Could you check a few things on this model? Use its own coordinates, in mm. Coordinates: 2 decimals unless noted, no trailing zeros. Loops run counter-clockwise (first coordinate to the right, second up) from the corner with the lowest first, then second, coordinate; pieces in that order, holes last. Notation, with made-up numbers: (19, 9) - (23, 9) arc R22 ccw to (23, 39) - close; hole circle Ø4 at (21, 57). An arc over 180 degrees is marked (long way). One line per item, written item: value. Start each with the question number.
(1) If I drill on line 1 along X through (y, z) = (1.8, 0); line 2 along X through (y, z) = (0.4, 85); line 3 along Z through (x, y) = (176, 2.3), over which ranges is the centre line in solid material (lowest first)? Write a range as from..to.
(2) If we section it at B-B on z = -17: Write out the boundary of the cut face in (x, y).
(3) If we section it at A-A on y = 2.5: Write out the boundary of the cut face in (x, z).
(4) If we section it at C-C on z = 63: Write out the boundary of the cut face in (x, y).
(5) I'm going to push a flat-ended pin straight in: P1, Ø4, axis at x = 202, z = 0, coming from the -Y side. Where does the tip first touch, or does it pass through?
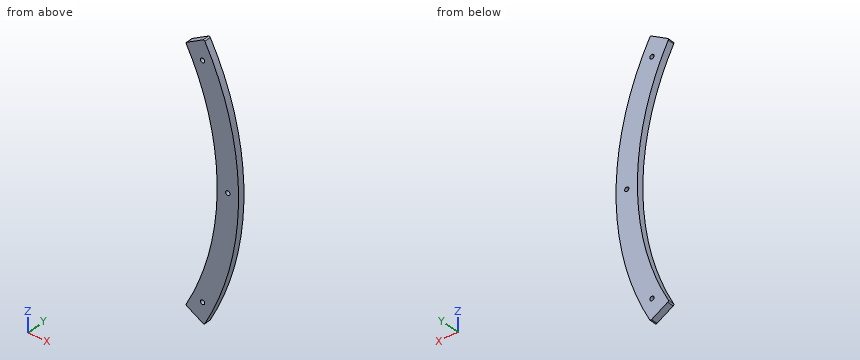
Autodesk Fusion 360 part; units mm, degrees
sketch "スケッチ1" plane through (0, 0, 0) normal (0, 1, 0) x (1, 0, 0)
  arc A0 (181.8653, -105) -> (181.8653, 105) centre (0, 0) ccw
  line L0 (181.8653, 105) -> (0, 0)
  line L1 (0, 0) -> (181.8653, -105)
  line L2 (0, 0) -> (210, 0)
  arc A1 (168.0089, -97) -> (168.0089, 97) centre (0, 0) ccw
  line L3 (10, 0) -> (184.3138, 100.6401)
  line L4 (10, 0) -> (184.3138, -100.6401)
  arc A2 (183.0742, -85.3689) -> (183.0742, 85.3689) centre (0, 0) ccw
  line L5 (0, 0) -> (183.0742, 85.3689)
  line L6 (0, 0) -> (183.0742, -85.3689)
  point P0 (202, 0)
  dimension "d1" = 210
  dimension "d2" = 30
  dimension "d3" = 30
  dimension "d4" = 194
  dimension "d14" = 30
  dimension "d15" = 10
  dimension "d17" = 30
  dimension "d23" = 202
  dimension "d24" = 25
  dimension "d25" = 25
extrude "押し出し1" add sketch "スケッチ1" along normal blind 5 contours A0 L2 A1 L4 A2 L6 | A0 L2 A1 L3 A2 L5 | L2 A1 A2 L6 | L2 A1 A2 L5
hole "穴1" at (183.0742, 0, 85.3689) at (202, 0, 0) at (183.0742, 0, -85.3689) direction (0, 1, 0) diameter 3.2 end through all
fillet "フィレット1" radius 1 4 edges at (184.3138, 2.5, 100.6401) (184.3138, 2.5, -100.6401) (170.4531, 2.5, 92.6377) (170.4531, 2.5, -92.6377)
Values:
1. line 1: x = 194..200.4, 203.6..210
1. line 2: x = 174.39..181.52, 184.63..192.03
1. line 3: z = -95.84..-81.61, 81.61..95.84
2. outline: (193.25, 0) - (209.31, 0) - (209.31, 5) - (193.25, 5) - close
3. outline: (170.91, -91.78) arc R1 ccw to (171.29, -93.12) - (183.42, -100.13) arc R1 ccw to (184.8, -99.74) arc R210 ccw to (184.8, 99.74) arc R1 ccw to (183.42, 100.13) - (171.29, 93.12) arc R1 ccw to (170.91, 91.78) arc R194 cw to start; hole circle Ø3.2 at (183.07, -85.37); hole circle Ø3.2 at (183.07, 85.37); hole circle Ø3.2 at (202, 0)
4. outline: (183.49, 0) - (200.33, 0) - (200.33, 5) - (183.49, 5) - close
5. P1: stops at y = 0
